Work out the finished part from the listing and answer in its coordinate system (mm). A direction names the side the tool comes from. Give positions to 0.01 mm unless a question says otherwise; leave off trailing zeros. Loops run counter-clockwise (first coordinate to the right, second up) from the corner with the lowest first, then second, coordinate; pieces in that order, holes last.
from build123d import *

# Parameters (mm, degrees)
SKETCH_1_R          = 7.5
EXTRUDE_1_DEPTH     = 6
SKETCH_2_R          = 6
CUT_EXTRUDE_1_DEPTH = 3


with BuildPart() as part:
    # 스케치1 → 보스-돌출1 (new body)
    with BuildSketch(Plane.XY):
        Circle(SKETCH_1_R)
    extrude(amount=EXTRUDE_1_DEPTH)

    # 스케치2 → 컷-돌출1 (cut)
    with BuildSketch(Plane.XY.offset(6)):
        Circle(SKETCH_2_R)
    extrude(amount=-CUT_EXTRUDE_1_DEPTH, mode=Mode.SUBTRACT)

    # 스케치8 → M2 소켓 머리 캡 나사용 카운터보어2 (revolve, cut)
    with BuildSketch(Plane.YZ):
        Polygon((0, 0), (0, 5.721032743), (1.2, 5), (1.2, 2), (2.25, 2), (2.25, 0.025), (2.275, 0), align=None)
    revolve(axis=Axis((0, 0, -6.35), (0, 0, 1)), mode=Mode.SUBTRACT)


solid = part.part
Item 1: For faces 1 (the face through (-2.23, -0.29, 1)), 2 (the face through (-0.1, 1.4, 3)), 3 (the face through (2, 2, 0)), determine the directions among +Z, -Z, +X, -X, +Y, -Y from which every point of the face is accessible in a straight line to the end or side of a thin tool.
Item 2: Find section D-D, the plane x = -3.75. Write down the section's boundary in (y, z).
Item 3: Find section C-C, the plane y = 4. Write down the section's boundary in (x, z), plus the area to 3 significant figures.
Item 4: Flat-ended cylindrical pins translate along their axes: pin 1 Ø1.5 at (x, z) = (4, 3.5) entering from +Y; pin 2 Ø5 at (x, y) = (0, 0) entering from +Z; pin 3 Ø4 at (x, y) = (0, 0) entering from -Z. Find the tip coordinate at first contact, or state that the pin passes through.
Item 5: Find section A-A, the plane x = 0. Write down the section's boundary in (y, z) (3 decimals).
Item 6: Consider line 1 (Y direction, x = 0, z = 5.4); line 2 (Y direction, x = 0, z = 2.55); line 3 (Z direction, x = 3.25, y = -1.75). Determine where each line is inside the solid, lowest interval first.
Item 7: Determine the mould class of faces 4 (the face through (2, 6, 6)), 5 (the face through (-7.493, 0.33, 2.958)), 6 (the face through (-6, 0, 5)), 7 (the face through (1, -1, 2)) for opening direction X: released by +X, released by -X, zero draft, split by the parting line, or undercut.
Ans:
1. face 1: -Z
1. face 2: +Z
1. face 3: -Z, +X, -X, +Y, -Y
2. outline: (-6.5, 0) - (6.5, 0) - (6.5, 6) - (4.68, 6) - (4.68, 3) - (-4.68, 3) - (-4.68, 6) - (-6.5, 6) - close
3. outline: (-6.34, 0) - (6.34, 0) - (6.34, 6) - (4.47, 6) - (4.47, 3) - (-4.47, 3) - (-4.47, 6) - (-6.34, 6) - close
3. area: 49.3 mm2
4. pin 1: stops at y = 6.76
4. pin 2: stops at z = 3
4. pin 3: stops at z = 2
5. outline: (-7.5, 0) - (-2.275, 0) - (-2.25, 0.025) - (-2.25, 2) - (-1.2, 2) - (-1.2, 3) - (-6, 3) - (-6, 6) - (-7.5, 6) - close; (1.2, 2) - (2.25, 2) - (2.25, 0.025) - (2.275, 0) - (7.5, 0) - (7.5, 6) - (6, 6) - (6, 3) - (1.2, 3) - close
6. line 1: y = -7.5 to -6, 6 to 7.5
6. line 2: y = -7.5 to -1.2, 1.2 to 7.5
6. line 3: z = 0 to 3
7. face 4: zero draft
7. face 5: split by the parting line
7. face 6: undercut
7. face 7: undercut
